Read the model definition and answer for the solid it produces. Units are mm, in the model's axes. Round coordinates to 2 decimals unless told otherwise and drop trailing zeros. Order: outer loops, then holes, each group sorted by start corner. A loop starts at its lowest first (then second) coordinate and runs counter-clockwise, first axis right, second up.
from build123d import *

# Parameters (mm, degrees)
SKETCH1_R           = 16
SKETCH1_R_2         = 1.6
BOSS_EXTRUDE1_DEPTH = 3
CHAMFER1_SIZE       = 1.2
FILLET1_R           = 0.5


with BuildPart() as part:
    # Sketch1 → Boss-Extrude1 (new body)
    with BuildSketch(Plane(origin=(0, 0, 0), x_dir=(1, 0, 0), z_dir=(0, 1, 0))):
        with Locations(Location((27.13838664, -2.073844751, 0), (0, 0, 270))):
            Circle(SKETCH1_R)
        with Locations(Location((23.771761103, 10.379099981, 0), (0, 0, 270))):
            Circle(SKETCH1_R_2, mode=Mode.SUBTRACT)
        with Locations(Location((36.239640361, 7.068210855, 0), (0, 0, 270))):
            Circle(SKETCH1_R_2, mode=Mode.SUBTRACT)
        with Locations(Location((39.606265898, -5.384733876, 0), (0, 0, 270))):
            Circle(SKETCH1_R_2, mode=Mode.SUBTRACT)
        with Locations(Location((30.505012177, -14.526789483, 0), (0, 0, 270))):
            Circle(SKETCH1_R_2, mode=Mode.SUBTRACT)
        with Locations(Location((18.037132919, -11.215900357, 0), (0, 0, 270))):
            Circle(SKETCH1_R_2, mode=Mode.SUBTRACT)
        with Locations(Location((14.670507382, 1.237044374, 0), (0, 0, 270))):
            Circle(SKETCH1_R_2, mode=Mode.SUBTRACT)
    extrude(amount=BOSS_EXTRUDE1_DEPTH)

    # Chamfer1
    chamfer1_edges = [part.edges().sort_by_distance(p)[0] for p in [
        (39.606265898, 3, 3.784733876),
        (30.505012177, 3, 12.926789483),
        (18.037132919, 3, 9.615900357),
        (14.670507382, 3, -2.837044374),
        (23.771761103, 3, -11.979099981),
        (36.239640361, 3, -8.668210855),
    ]]
    chamfer(chamfer1_edges, length=CHAMFER1_SIZE)

    # Fillet1
    # the kernel refuses this fillet: 0.5 mm, written as the material it takes off along each edge
    with BuildSketch(Plane(origin=(27.13838664, 3, 2.073844751), x_dir=(0, 0, 1), z_dir=(-1, 0, 0))) as fillet1_piece_1:
        with BuildLine():
            CenterArc((16 - FILLET1_R, -FILLET1_R), FILLET1_R, 0, 90)
            Line((16, -FILLET1_R), (16, 0))
            Line((16, 0), (16 - FILLET1_R, 0))
        make_face()
    revolve(axis=Axis((27.13838664, 3, 2.073844751), (0, 1, 0)), mode=Mode.SUBTRACT)


solid = part.part
Q1. A cutting plane is placed at A-A, the plane y = 1.35. Give the vertices of the cut face in (x, z).
Outcome:
outline: circle Ø32 at (27.14, 2.07); hole circle Ø3.2 at (14.67, -1.24); hole circle Ø3.2 at (18.04, 11.22); hole circle Ø3.2 at (23.77, -10.38); hole circle Ø3.2 at (30.51, 14.53); hole circle Ø3.2 at (36.24, -7.07); hole circle Ø3.2 at (39.61, 5.38)
Q2. For a pull along Z with two mould halves and no side action, classify faces 1 (the face through (11.519, 1.232, -1.395)), 2 (the face through (27, 3, 2)), 3 (the face through (31.85, 0.89, 15.39)) as released by +Z, released by -Z, zero draft, split by the parting line, or undercut.
Outcome:
face 1: split by the parting line
face 2: zero draft
face 3: undercut
Q3. Flat-ended cylindrical pins translate along their axes: pin 1 (2.5 mm diameter, centred on x = 39.61, z = 5.38, fed in from -Y); pin 2 (1 mm diameter, centred on y = 0.5, z = 13.5, fed in from -X); pin 3 (5 mm diameter, centred on x = 18.04, z = 11.22, fed in from +Y) (3 decimals). Find the tip coordinate at first contact, or state that the pin passes through.
Outcome:
pin 1: passes through
pin 2: stops at x = 15.45
pin 3: stops at y = 2.705
Q4. Straight lines are drawn through the part: probe 1 along X at (y, z) = (0.6, -2); probe 2 along Z at (x, y) = (32, 2.45); probe 3 along X at (y, z) = (0.5, -8). For each, find the intervals that lie inside material, in ascending order.
Outcome:
probe 1: x = 11.67 to 13.26, 16.08 to 42.61
probe 2: z = -13.17 to 12.85, 16.21 to 17.32
probe 3: x = 14.71 to 34.94, 37.54 to 39.57
